Here's how the part is built. I have some questions about the finished solid (model axes, mm). A direction names the side the tool comes from. Coordinates: 2 decimals unless noted, no trailing zeros. Order: outer loops, then holes, each group sorted by start corner. A loop starts at its lowest first (then second) coordinate and runs counter-clockwise, first axis right, second up.
```python
from build123d import *

# Parameters (mm, degrees)
SKETCH_R        = 4.1
SKETCH_R_2      = 2.55
PAD_DEPTH       = 8
SKETCH001_W     = 15
SKETCH001_H     = 15
POCKET_DEPTH    = 2.5
SKETCH002_W     = 15
SKETCH002_H     = 15
POCKET001_DEPTH = 2.5
SKETCH003_R     = 1
POCKET002_DEPTH = 7
FILLET_R        = 2


with BuildPart() as part:
    # Sketch → Pad (new body)
    with BuildSketch(Plane.XY):
        with BuildLine():
            ThreePointArc((7.986353, -6.983084), (14.5, 0), (7.986353, 6.983084))
            Line((-9.28, 4.132989), (7.986353, 6.983084))
            ThreePointArc((-9.28, 4.132989), (-12, 0), (-9.28, -4.132989))
            Line((-9.28, -4.132989), (7.986353, -6.983084))
        make_face()
        with Locations((7.5, 0)):
            Circle(SKETCH_R, mode=Mode.SUBTRACT)
        with Locations((-7.5, 0)):
            Circle(SKETCH_R_2, mode=Mode.SUBTRACT)
    extrude(amount=PAD_DEPTH)

    # Sketch001 (on Face8 of Pad) → Pocket (cut)
    with BuildSketch(Plane.XY.offset(8)):
        with Locations((-6, 0)):
            Rectangle(SKETCH001_W, SKETCH001_H)
    extrude(amount=-POCKET_DEPTH, mode=Mode.SUBTRACT)

    # Sketch002 (on Face4 of Pocket) → Pocket001 (cut)
    with BuildSketch(Plane(origin=(0, 0, 0), x_dir=(1, 0, 0), z_dir=(0, 0, -1))):
        with Locations((-6, 0)):
            Rectangle(SKETCH002_W, SKETCH002_H)
    extrude(amount=-POCKET001_DEPTH, mode=Mode.SUBTRACT)

    # Sketch003 → Pocket002 (cut)
    with BuildSketch(Plane.XZ):
        with Locations((7.5, 4.15)):
            Circle(SKETCH003_R)
    extrude(amount=-POCKET002_DEPTH, mode=Mode.SUBTRACT)

    # Fillet
    fillet_edges = [part.edges().sort_by_distance(p)[0] for p in [
        (-9.28, 4.132989, 4),
        (7.986353, 6.983084, 6.511881),
        (7.986353, 6.983084, 1.638119),
        (7.986353, -6.983084, 4),
        (-9.28, -4.132989, 4),
    ]]
    fillet(fillet_edges, radius=FILLET_R)


solid = part.part
```
Q1. I need wall thicknesses on L1, parallel to X at y = -1.5, z = 3.5; L2, parallel to Z at x = 7.5, y = 6.2; L3, parallel to Z at x = -4, y = 4.5. Which ranges of each line are inside material? Lowest first, please.
Q2. If we section it at A-A on y = 0: Write out the boundary of the cut face in (x, z).
Q3. For faces 4 (the flat face through (1.5, 0, 7)), 5 (the cylindrical face through (8.454, 5.449, 4.45)), 6 (the flat face through (1.5, 0, 1)), which set-ups out of +Z, -Z, +X, -X, +Y, -Y let a thin tool reach every point of the face, with its end or its side?
Q4. If we section it at C-C on x = 7.25: Write out the boundary of the cut face in (y, z), then the cut area to 3 significant figures.
Q5. Will these pins go through, and if not, where does the flat tip stop? pin 1 (1.6 mm diameter, centred on x = 7.5, z = 4.15, fed in from +Y); pin 2 (1 mm diameter, centred on y = -3, z = 1, fed in from +X); pin 3 (1.2 mm diameter, centred on y = 0.5, z = 2, fed in from -X); pin 4 (5 mm diameter, centred on x = 11.5, y = -2, fed in from -Z).
Q6. We'd pull the mould along X, two halves only. Please class faces 1 (the cylindrical face through (-12, 0, 4)), 2 (the cylindrical face through (-5.144, -0.977, 3.979)), 3 (the flat face through (-4, 0, 5.5)): pulls with the +X half, pulls with the -X half, needs draft (parallel to the pull), parting line crosses it, or undercut.
Q7. If we section it at B-B on z = 7: Write out the boundary of the cut face in (x, y), then the cut area to 3 significant figures.
Q8. If we section it at D-D on y = -3.5: Write out the boundary of the cut face in (x, z).
Reply:
1. L1: x = -11.74 to -9.56, -5.44 to 3.68, 11.32 to 14.34
1. L2: z = 0 to 3.15, 5.15 to 8
1. L3: z = 2.5 to 5.5
2. outline: (-12, 2.5) - (-10.05, 2.5) - (-10.05, 5.5) - (-12, 5.5) - close; (-4.95, 2.5) - (1.5, 2.5) - (1.5, 0) - (3.4, 0) - (3.4, 8) - (1.5, 8) - (1.5, 5.5) - (-4.95, 5.5) - close; (11.6, 0) - (14.5, 0) - (14.5, 8) - (11.6, 8) - close
3. face 4: +Z, -X, +Y, -Y
3. face 5: +Y
3. face 6: -Z, -X, +Y, -Y
4. outline: (-6.86, 0) - (-4.09, 0) - (-4.09, 8) - (-6.86, 8) - close; (4.09, 0) - (6.86, 0) - (6.86, 3.18) - (4.09, 3.18) - close; (4.09, 5.12) - (6.86, 5.12) - (6.86, 8) - (4.09, 8) - close
4. area: 38.9 mm2
5. pin 1: stops at y = -4.02
5. pin 2: stops at x = 14.04
5. pin 3: stops at x = -12
5. pin 4: stops at z = 0
6. face 1: pulls with the -X half
6. face 2: undercut
6. face 3: needs draft
7. outline: (1.5, -5.91) - (7.74, -6.94) arc R2 ccw to (8.29, -6.96) arc R7 ccw to (8.29, 6.96) arc R2 ccw to (7.74, 6.94) - (1.5, 5.91) - close; hole circle Ø8.2 at (7.5, 0)
7. area: 101 mm2
8. outline: (-10.33, 2.5) - (1.5, 2.5) - (1.5, 0) - (5.36, 0) - (5.36, 8) - (1.5, 8) - (1.5, 5.5) - (-10.33, 5.5) - close; (9.64, 0) - (13.56, 0) - (13.56, 8) - (9.64, 8) - close
